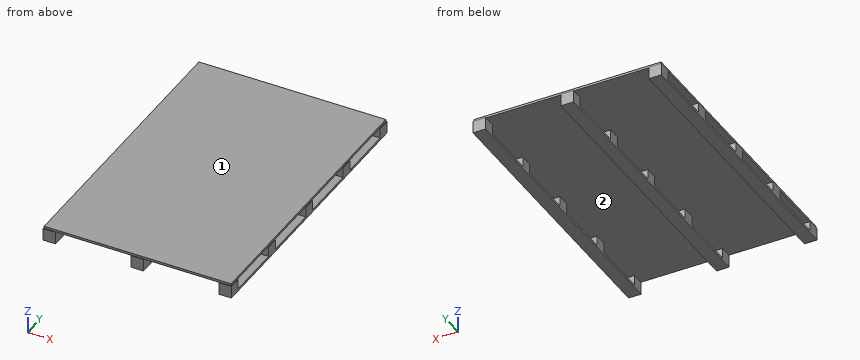
```python
from build123d import *

# Parameters (mm, degrees)
F0_W     = 1488
F0_H     = 2288
F1_DEPTH = 18
F2_W     = 100
F2_H     = 100
F3_DEPTH = 80
F4_W     = 100
F4_H     = 2300
F5_DEPTH = 18


with BuildPart() as f1:
    # F0 (on Top) → F1 (new body)
    with BuildSketch(Plane.XY):
        Rectangle(F0_W, F0_H)
    extrude(amount=F1_DEPTH)

    # F2 (on face) → F3 (join)
    with BuildSketch(Plane(origin=(0, 0, 0), x_dir=(1, 0, 0), z_dir=(0, 0, -1))):
        with Locations((-700, 1100)):
            Rectangle(F2_W, F2_H)
        with Locations((-700, 550)):
            Rectangle(F2_W, F2_H)
        with Locations((-700, 0)):
            Rectangle(F2_W, F2_H)
        with Locations((-700, -550)):
            Rectangle(F2_W, F2_H)
        with Locations((-700, -1100)):
            Rectangle(F2_W, F2_H)
        with Locations((0, 1100)):
            Rectangle(F2_W, F2_H)
        with Locations((0, 550)):
            Rectangle(F2_W, F2_H)
        Rectangle(F2_W, F2_H)
        with Locations((0, -550)):
            Rectangle(F2_W, F2_H)
        with Locations((0, -1100)):
            Rectangle(F2_W, F2_H)
        with Locations((700, 1100)):
            Rectangle(F2_W, F2_H)
        with Locations((700, 550)):
            Rectangle(F2_W, F2_H)
        with Locations((700, 0)):
            Rectangle(F2_W, F2_H)
        with Locations((700, -550)):
            Rectangle(F2_W, F2_H)
        with Locations((700, -1100)):
            Rectangle(F2_W, F2_H)
    extrude(amount=F3_DEPTH)

    # F4 (on face) → F5 (join)
    with BuildSketch(Plane(origin=(0, 0, -80), x_dir=(1, 0, 0), z_dir=(0, 0, -1))):
        with Locations((-700, 0)):
            Rectangle(F4_W, F4_H)
        Rectangle(F4_W, F4_H)
        with Locations((700, 0)):
            Rectangle(F4_W, F4_H)
    extrude(amount=F5_DEPTH)


solid = f1.part
```
The model under review builds one solid part; all positions refer to its coordinate system, in mm. Face numbers are marked on the shaded views. Round coordinates to 2 decimals unless told otherwise and drop trailing zeros. Order: outer loops, then holes, each group sorted by start corner. A loop starts at its lowest first (then second) coordinate and runs counter-clockwise, first axis right, second up.
(1) Take a section at A-A, the plane y = 120. State the section outline as (x, z) points.
Working result:
outline: (-750, -98) - (-650, -98) - (-650, -80) - (-750, -80) - close; (-744, 0) - (744, 0) - (744, 18) - (-744, 18) - close; (-50, -98) - (50, -98) - (50, -80) - (-50, -80) - close; (650, -98) - (750, -98) - (750, -80) - (650, -80) - close
(2) Wall thickness on L1, parallel to X at y = 191.5, z = -84; L2, parallel to Y at x = -26, z = -30.5; L3, parallel to Z at x = 8.5, y = 266: over which ranges is each line inside the solid? List them lowest first.
Working result:
L1: x = -750 to -650, -50 to 50, 650 to 750
L2: y = -1150 to -1050, -600 to -500, -50 to 50, 500 to 600, 1050 to 1150
L3: z = -98 to -80, 0 to 18
(3) Mouldability with a two-part tool opening along Y and no side actions: class the marked faces 1 and 2 as released by +Y, released by -Y, zero draft, split by the parting line, or undercut.
Working result:
face 1: zero draft
face 2: undercut
(4) Take a section at C-C, the plane x = -549. State the section outline as (y, z) points, plus the area to 3 significant figures.
Working result:
outline: (-1144, 0) - (1144, 0) - (1144, 18) - (-1144, 18) - close
area: 41,200 mm2
(5) Take a section at B-B, the plane z = -62.5. Count the separate pieces of the cut face and the enclosed holes in it, plus the area to 3 significant figures.
Working result:
separate pieces: 15
enclosed holes: 0
area: 150,000 mm2
(6) For P1, Ø1.8, axis at x = -747, y = -547, coming from the +Z side; P2, Ø10, axis at x = -219.5, y = -711, coming from the -Z side; P3, Ø20, axis at y = 476, z = 12.5, coming from the +X side, all flat-tipped, find the tip position at first contact; note any pin that passes through.
Working result:
P1: stops at z = 0
P2: stops at z = 0
P3: stops at x = 744
